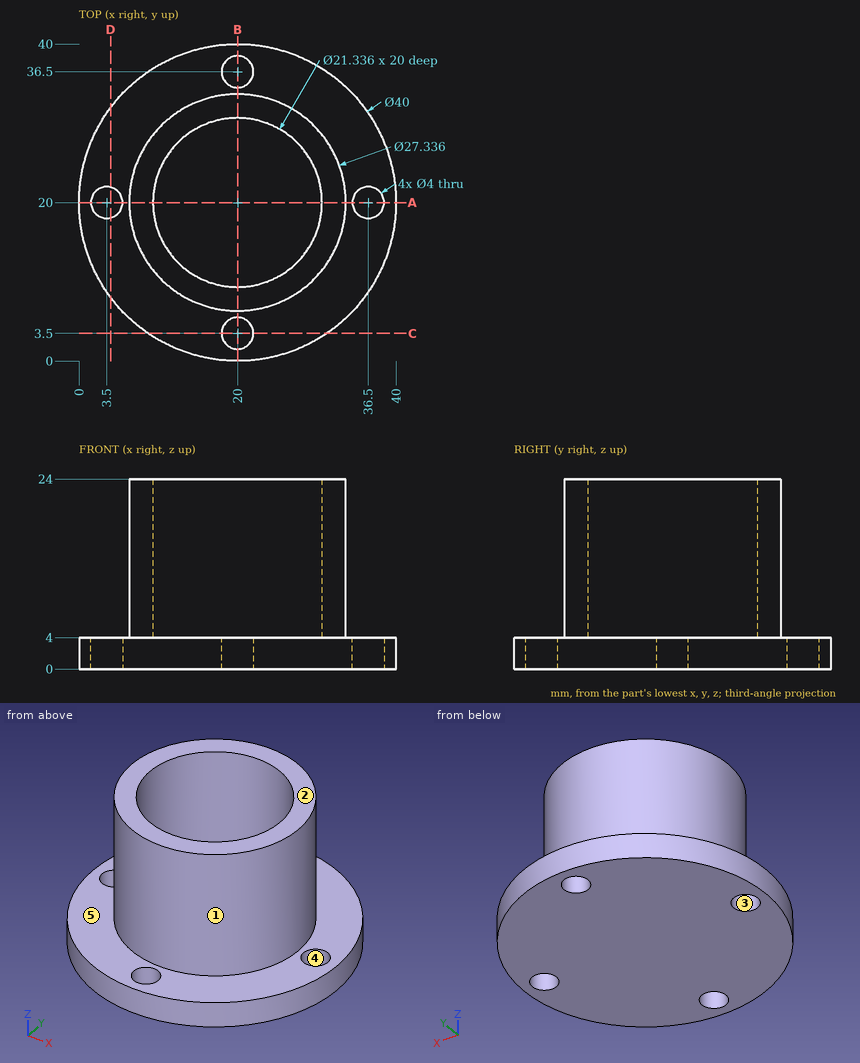
Answer from the drawing. Dimensions are ordinates in mm from the lowest x, y and z of the part. A direction names the side the tool comes from. Round coordinates to 2 decimals unless told otherwise and drop trailing zeros. Loops run counter-clockwise (first coordinate to the right, second up) from the corner with the lowest first, then second, coordinate; pieces in that order, holes last. Notation, with made-up numbers: (-39.75, 19) - (4.25, 19) arc R18 ccw to (4.25, 28) - close; hole circle Ø8 at (31, 68). An arc over 180 degrees is marked (long way). Return JSON: item names as keys, results as strings. Group by question number.
1. Which of the six approach directions +Z, -Z, +X, -X, +Y, -Y give full straight-line access (tool end or side, diameter ignored) to the marked faces 4 and 5?
2. The part is cut by section C-C on y = 3.5. Determine the outline of the cut face in (x, z).
3. The part is cut by section D-D on x = 4. Determine the outline of the cut face in (y, z).
4. Each of these flat-tipped pins is pushed along its axis until it touches: P1, Ø5, axis at x = 20, y = 36.5, coming from the +Z side; P2, Ø3, axis at x = 24, z = 12.5, coming from the -Y side; P3, Ø1.5, axis at x = 31.5, z = 7.5, coming from the -Y side. Where does it stop, or does it pass through?
5. The part is cut by section A-A on y = 20. Determine the outline of the cut face in (x, z), then the cut area to 3 significant figures.
6. The mould has two halves that part along Y. Classify the marked faces 1, 2 and 3: pulls with the +Y half, pulls with the -Y half, needs draft (parallel to the pull), parting line crosses it, or undercut.
7. Consider probe 1 along Y at (x, z) = (20, 2.5); probe 2 along Y at (x, z) = (20, 4.5); probe 3 along Z at (x, y) = (23, 19). Determine where each line is inside the solid, lowest interval first.
Resolved:
{
 "1": {"face 4": "+Z, -Z", "face 5": "+Z"},
 "2": {"outline": "(8.7, 0) - (18, 0) - (18, 4) - (8.7, 4) - close; (22, 0) - (31.3, 0) - (31.3, 4) - (22, 4) - close"},
 "3": {"outline": "(8, 0) - (18.06, 0) - (18.06, 4) - (8, 4) - close; (21.94, 0) - (32, 0) - (32, 4) - (21.94, 4) - close"},
 "4": {"P1": "stops at z = 4", "P2": "stops at y = 6.56", "P3": "stops at y = 11.56"},
 "5": {"outline": "(0, 0) - (1.5, 0) - (1.5, 4) - (0, 4) - close; (5.5, 0) - (34.5, 0) - (34.5, 4) - (33.67, 4) - (33.67, 24) - (30.67, 24) - (30.67, 4) - (9.33, 4) - (9.33, 24) - (6.33, 24) - (6.33, 4) - (5.5, 4) - close; (38.5, 0) - (40, 0) - (40, 4) - (38.5, 4) - close", "area": "248 mm²"},
 "6": {"face 1": "parting line crosses it", "face 2": "needs draft", "face 3": "undercut"},
 "7": {"probe 1": "y = 0 to 1.5, 5.5 to 34.5, 38.5 to 40", "probe 2": "y = 6.33 to 9.33, 30.67 to 33.67", "probe 3": "z = 0 to 4"}
}
